Input: part model. Units: mm. Frame: model coordinates. Coordinates: 2 decimals unless noted, no trailing zeros. Loops run counter-clockwise (first coordinate to the right, second up) from the corner with the lowest first, then second, coordinate; pieces in that order, holes last. Notation, with made-up numbers: (15.25, 15.25) - (66.25, 15.25) arc R5 ccw to (66.25, 24.25) - close; hole circle Ø8 at (7, -1). An arc over 180 degrees is marked (long way). Answer as CSV lines item,"result". Start each with the question number.
```python
from build123d import *

# Parameters (mm, degrees)
F0_R     = 42.633401
F1_DEPTH = 190.5
F2_R     = 42.311507
F3_R     = 41.698297


with BuildPart() as f1:
    # F0 (on Right) → F1 (new body)
    with BuildSketch(Plane.YZ):
        Circle(F0_R)
    extrude(amount=F1_DEPTH)

    # F2
    f2_edges = [f1.edges().sort_by_distance(p)[0] for p in [
        (190.5, -42.633401, 0),
    ]]
    fillet(f2_edges, radius=F2_R)

    # F3
    f3_edges = [f1.edges().sort_by_distance(p)[0] for p in [
        (0, -42.633401, 0),
    ]]
    fillet(f3_edges, radius=F3_R)


solid = f1.part
```
Item 1: Section query A-A, the plane x = 61. Output: boundary loops of the cut face in (y, z), and give its area (3 significant figures).
Item 2: Material intervals for probe 1 along X at (y, z) = (2.5, -26.5); probe 2 along X at (y, z) = (-15.5, -24); probe 3 along Y at (x, z) = (27, -35), sorted ascending.
Item 3: Contact query for flat-ended pins moving along their axis: P1, Ø10, axis at x = 123.5, y = -4, coming from the +Z side; P2, Ø10, axis at x = 103, z = -26.5, coming from the -Y side; P3, Ø5, axis at x = 42.5, z = 10.5, coming from the -Y side. Output: stop coordinate, or through.
Response values:
1,outline,"circle Ø85.27 at (0, 0)"
1,area,"5,710 mm²"
2,probe 1,"x = 8.85 to 181.34"
2,probe 2,"x = 10.47 to 179.69"
2,probe 3,"y = -19.28 to 19.28"
3,P1,"stops at z = 42.63"
3,P2,"stops at y = -36.82"
3,P3,"stops at y = -41.88"
